Read the model definition and answer for the solid it produces. Units are mm, in the model's axes. Face numbers are marked on the shaded views. A direction names the side the tool comes from. Give positions to 0.01 mm unless a question says otherwise; leave off trailing zeros. Write each loop counter-clockwise with the first axis right and the second up, starting at its lowest first coordinate (ties: lowest second). Pieces come first, ordered by that corner, then holes. Notation, with made-up numbers: (-27.75, 18.5) -> (-19.75, 18.5) arc R28 ccw to (-19.75, 40.5) -> close; hole circle Ø7 at (73, -24). An arc over 180 degrees is marked (long way). Answer as CSV lines item,"result". Start each with the question number.
1. A tool of negligible diameter and unlimited length cuts with its end or side. For the marked faces 1, 2 and 3, from which of +Z, -Z, +X, -X, +Y, -Y can it reach the whole face along a straight path? Write none if from no direction.
2. The part is cut by section C-C, the plane y = 1. Determine the outline of the cut face in (x, z).
3. Given pin 1 (2 mm diameter, centred on x = 6, y = 0.5, fed in from -Z); pin 2 (1.5 mm diameter, centred on y = 2.5, z = 3.5, fed in from +X); pin 3 (2 mm diameter, centred on x = -10.5, z = 3.5, fed in from +Y), each flat-ended and moving along its own axis, determine where each tip first touches the part or whether it passes through.
4. Find the intervals of material crossed by line 1 (Y direction, x = 6, z = 2.35); line 2 (X direction, y = -0.25, z = 4.6); line 3 (X direction, y = 1, z = 3), in increasing order.
5. The part is cut by section A-A, the plane x = -5.5. Determine the outline of the cut face in (y, z).
6. The part is cut by section D-D, the plane y = -0.25. Determine the outline of the cut face in (x, z).
7. The part is cut by section B-B, the plane z = 2.2. Give the number of separate pieces and of enclosed holes in the cut face, and give its area (3 significant figures).
8. For a pull along X with two mould halves and no side action, classify the marked faces 4, 5 and 6 as pulls with the +X half, pulls with the -X half, needs draft (parallel to the pull), parting line crosses it, or undercut.
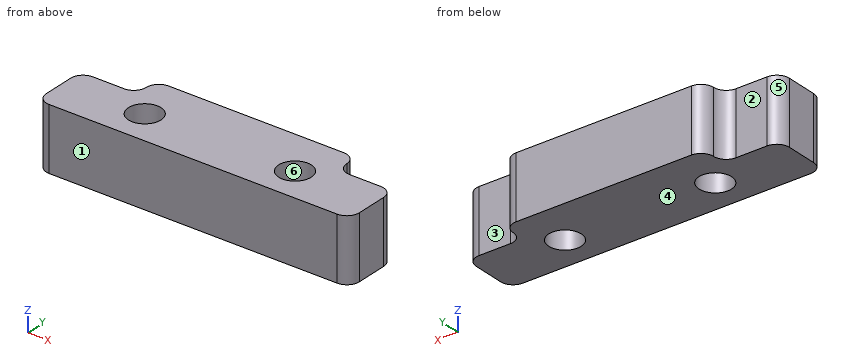
from build123d import *

# Parameters (mm, degrees)
SKETCH_1_R      = 1.3
EXTRUDE_1_DEPTH = 5
FILLET_1_R      = 1


with BuildPart() as part:
    # 草图1 → 凸台-拉伸1 (new body)
    with BuildSketch(Plane.XY):
        Polygon((12.5, -2.25), (-12.5, -2.25), (-12.5, 2.25), (-8, 2.25), (-8, 4.25), (8, 4.25), (8, 2.25), (12.5, 2.25), align=None)
        with Locations((-6, 0.5)):
            Circle(SKETCH_1_R, mode=Mode.SUBTRACT)
        with Locations(Location((6, 0.5, 0), (0, 0, 180))):
            Circle(SKETCH_1_R, mode=Mode.SUBTRACT)
    extrude(amount=EXTRUDE_1_DEPTH)

    # 圆角1
    fillet_1_edges = [part.edges().sort_by_distance(p)[0] for p in [
        (12.5, -2.25, 2.5),
        (12.5, 2.25, 2.5),
        (-12.5, -2.25, 2.5),
        (-12.5, 2.25, 2.5),
        (-8, 4.25, 2.5),
        (8, 4.25, 2.5),
        (8, 2.25, 2.5),
        (-8, 2.25, 2.5),
    ]]
    fillet(fillet_1_edges, radius=FILLET_1_R - 0.0001)  # a hair under: the kernel refuses the full size


solid = part.part
Results found:
1,face 1,"+Z, -Z, +X, -X, -Y"
1,face 2,"+Z, -Z, -X, +Y"
1,face 3,"+Z, -Z, +X, +Y"
2,outline,"(-12.5, 0) -> (-7.2, 0) -> (-7.2, 5) -> (-12.5, 5) -> close; (-4.8, 0) -> (4.8, 0) -> (4.8, 5) -> (-4.8, 5) -> close; (7.2, 0) -> (12.5, 0) -> (12.5, 5) -> (7.2, 5) -> close"
3,pin 1,"passes through"
3,pin 2,"stops at x = 12.37"
3,pin 3,"stops at y = 2.25"
4,line 1,"y = -2.25 to -0.8, 1.8 to 4.25"
4,line 2,"x = -12.5 to -7.06, -4.94 to 4.94, 7.06 to 12.5"
4,line 3,"x = -12.5 to -7.2, -4.8 to 4.8, 7.2 to 12.5"
5,outline,"(-2.25, 0) -> (-0.7, 0) -> (-0.7, 5) -> (-2.25, 5) -> close; (1.7, 0) -> (4.25, 0) -> (4.25, 5) -> (1.7, 5) -> close"
6,outline,"(-12.5, 0) -> (-7.06, 0) -> (-7.06, 5) -> (-12.5, 5) -> close; (-4.94, 0) -> (4.94, 0) -> (4.94, 5) -> (-4.94, 5) -> close; (7.06, 0) -> (12.5, 0) -> (12.5, 5) -> (7.06, 5) -> close"
7,separate pieces,"1"
7,enclosed holes,"2"
7,area,"133 mm²"
8,face 4,"needs draft"
8,face 5,"pulls with the -X half"
8,face 6,"undercut"
